from build123d import *

# Parameters (mm, degrees)
CYLINDER001_R     = 5
CYLINDER001_DEPTH = 3
CYLINDER_R        = 6
CYLINDER_DEPTH    = 2
CYLINDER005_R     = 1.5
CYLINDER005_DEPTH = 10
CYLINDER004_R     = 1.5
CYLINDER004_DEPTH = 10
CYLINDER003_R     = 1.5
CYLINDER003_DEPTH = 2
CYLINDER002_R     = 1.5
CYLINDER002_DEPTH = 2


with BuildPart() as cylinder001:
    # Cylinder001 → Cylinder001 (new body)
    with BuildSketch(Plane.XY):
        Circle(CYLINDER001_R)
    extrude(amount=CYLINDER001_DEPTH)


with BuildPart() as cut:
    # Cylinder → Cylinder (new body)
    with BuildSketch(Plane.XY):
        Circle(CYLINDER_R)
    extrude(amount=CYLINDER_DEPTH)

    # Cut: cut Cylinder001
    add(cylinder001.part, mode=Mode.SUBTRACT)


with BuildPart() as cylinder005:
    # Cylinder005 → Cylinder005 (new body)
    with BuildSketch(Plane(origin=(-1.25, 7, 0), x_dir=(1, 0, 0), z_dir=(0, 0, 1))):
        Circle(CYLINDER005_R)
    extrude(amount=CYLINDER005_DEPTH)


with BuildPart() as fusion:
    # Cylinder004 → Cylinder004 (new body)
    with BuildSketch(Plane(origin=(-7, 1.25, 0), x_dir=(1, 0, 0), z_dir=(0, 0, 1))):
        Circle(CYLINDER004_R)
    extrude(amount=CYLINDER004_DEPTH)

    # Fusion: union Cylinder005
    add(cylinder005.part)


with BuildPart() as cylinder003:
    # Cylinder003 → Cylinder003 (new body)
    with BuildSketch(Plane(origin=(0, 7, 0), x_dir=(1, 0, 0), z_dir=(0, 0, 1))):
        Circle(CYLINDER003_R)
    extrude(amount=CYLINDER003_DEPTH)


with BuildPart() as fusion002:
    # Cylinder002 → Cylinder002 (new body)
    with BuildSketch(Plane(origin=(-7, 0, 0), x_dir=(1, 0, 0), z_dir=(0, 0, 1))):
        Circle(CYLINDER002_R)
    extrude(amount=CYLINDER002_DEPTH)

    # Fusion001: union Cylinder003
    add(cylinder003.part)

    # Cut001: cut Fusion
    add(fusion.part, mode=Mode.SUBTRACT)

    # Fusion002: union Cut
    add(cut.part)


solid = fusion002.part
Design review of the part built by this model. Coordinates are the model's own, in mm. Coordinates: 2 decimals unless noted, no trailing zeros. Write each loop counter-clockwise with the first axis right and the second up, starting at its lowest first coordinate (ties: lowest second). Pieces come first, ordered by that corner, then holes. Notation, with made-up numbers: (31.25, 85) -> (80.25, 85) arc R18 ccw to (80.25, 92) -> close; hole circle Ø8 at (54.25, -30.5). An arc over 180 degrees is marked (long way). Write each question's results on one line, items separated by ' | '. Start each with the question number.
(1) The part is to be moulded in two halves that separate along X. For faces 1 (the face through (-7.9, -1.2, 1)), 2 (the face through (-5, 2, 2)), 3 (the face through (0.22, 7.29, 0.99)), say which applies: pulls with the +X half, pulls with the -X half, needs draft (parallel to the pull), parting line crosses it, or undercut.
(2) Take a section at C-C on z = 0.45. Write out the cut boundary in (x, y) (3 decimals).
(3) Take a section at B-B on y = 3.5. Write out the cut boundary in (x, z).
(4) For line 1 along Y through (x, z) = (0, 1.4); line 2 along X through (y, z) = (0, 1.05); line 3 along X through (y, z) = (-2.5, 1.25), list the stretches that pass through material, from the lowest coordinate up. Write a range as from..to.
(5) Clearance check with a flat-ended pin moving along its axis: P1, Ø1, axis at y = 6, z = 1, coming from the -X side. State where the tip first meets the part, or that it passes through.
(6) Take a section at A-A on x = -2. Write out the cut boundary in (y, z).
Results found:
1) face 1: undercut | face 2: needs draft | face 3: pulls with the -X half
2) outline: (-8.364, 0.625) arc R1.5 ccw to (-5.911, -1.031) arc R6 ccw (long way) to (1.031, 5.911) arc R1.5 ccw to (-0.625, 8.364) arc R1.5 cw to (-0.133, 5.999) arc R6 ccw to (-5.999, 0.133) arc R1.5 cw to start; hole circle Ø10 at (0, 0)
3) outline: (-4.87, 0) -> (-3.57, 0) -> (-3.57, 2) -> (-4.87, 2) -> close; (3.57, 0) -> (4.87, 0) -> (4.87, 2) -> (3.57, 2) -> close
4) line 1: y = -6..-5, 5..6.17, 7.83..8.5 | line 2: x = -8.5..-7.83, -6.17..-5, 5..6 | line 3: x = -5.45..-4.33, 4.33..5.45
5) P1: stops at x = -2.4
6) outline: (-5.66, 0) -> (-4.58, 0) -> (-4.58, 2) -> (-5.66, 2) -> close; (4.58, 0) -> (5.66, 0) -> (5.66, 2) -> (4.58, 2) -> close
